Part model, mm, in its own coordinate system. A direction names the side the tool comes from. Coordinates: 2 decimals unless noted, no trailing zeros. Loops run counter-clockwise (first coordinate to the right, second up) from the corner with the lowest first, then second, coordinate; pieces in that order, holes last.
```python
from build123d import *

# Parameters (mm, degrees)
CROQUIS1_R              = 2.4
SALIENTE_EXTRUIR1_DEPTH = 6
CROQUIS2_R              = 3.5
SALIENTE_EXTRUIR2_DEPTH = 1
CROQUIS3_R              = 18.5
SALIENTE_EXTRUIR3_DEPTH = 3
CORTAR_EXTRUIR1_DEPTH   = 2
CROQUIS5_R              = 2.075
CORTAR_EXTRUIR2_DEPTH   = 2.2
CROQUIS6_R              = 1.25
CORTAR_EXTRUIR3_DEPTH   = 28.300915736


with BuildPart() as part:
    # Croquis1 → Saliente-Extruir1 (new body)
    with BuildSketch(Plane.XY):
        Circle(CROQUIS1_R)
    extrude(amount=SALIENTE_EXTRUIR1_DEPTH)

    # Croquis2 → Saliente-Extruir2 (add)
    with BuildSketch(Plane(origin=(0, 0, 0), x_dir=(-1, 0, 0), z_dir=(0, 0, -1))):
        Circle(CROQUIS2_R)
    extrude(amount=SALIENTE_EXTRUIR2_DEPTH)

    # Croquis3 → Saliente-Extruir3 (add)
    with BuildSketch(Plane(origin=(0, 0, -1), x_dir=(-1, 0, 0), z_dir=(0, 0, -1))):
        Circle(CROQUIS3_R)
    extrude(amount=SALIENTE_EXTRUIR3_DEPTH)

    # Croquis4 → Cortar-Extruir1 (cut)
    with BuildSketch(Plane(origin=(0, 0, -4), x_dir=(-1, 0, 0), z_dir=(0, 0, -1))):
        with BuildLine():
            Line((0, 15.331093131), (-1.68173019, 12.418250997))
            ThreePointArc((-1.68173019, 12.418250997), (-1.649800286, 12.176683613), (-1.408167444, 12.145252908))
            ThreePointArc((-1.408167444, 12.145252908), (-0.72912408, 12.427844555), (0, 12.524467551))
            ThreePointArc((0, 12.524467551), (0.72912408, 12.427844555), (1.408167444, 12.145252908))
            ThreePointArc((1.408167444, 12.145252908), (1.649800286, 12.176683613), (1.68173019, 12.418250997))
            Line((1.68173019, 12.418250997), (0, 15.331093131))
        make_face()
    extrude(amount=-CORTAR_EXTRUIR1_DEPTH, mode=Mode.SUBTRACT)

    # Croquis5 → Cortar-Extruir2 (cut)
    with BuildSketch(Plane.XY.offset(6)):
        Circle(CROQUIS5_R)
    extrude(amount=-CORTAR_EXTRUIR2_DEPTH, mode=Mode.SUBTRACT)

    # Croquis6 → Cortar-Extruir3 (cut, through all)
    with BuildSketch(Plane.XY.offset(3.8)):
        Circle(CROQUIS6_R)
    extrude(amount=-CORTAR_EXTRUIR3_DEPTH, mode=Mode.SUBTRACT)


solid = part.part
```
Q1. Saw through at D-D (x = 5.5). List the corners of the cut face in (y, z), plus the area to 3 significant figures.
Q2. Probe line 1 (Y direction, x = 0, z = 4.7) (3 decimals); line 2 (Y direction, x = 0, z = 1.5); line 3 (Z direction, x = 2.5, y = -15.5). List the from-to ranges inside material, lowest first.
Q3. Saw through at A-A (y = 0). List the corners of the cut face in (x, z) (3 decimals).
Q4. Tool access for faces 1 (the flat face through (0.829, 13.895, -3.014)), 2 (the cylindrical face through (-0.27, -1.22, -0.05)), 3 (the cylindrical face through (1.29, 2.024, 2.958)): list every direction of +Z, -Z, +X, -X, +Y, -Y with a clear straight run to the whole face (end or side of a thin tool).
Q5. Drop flat-ended pins along their axis: P1, Ø1.5, axis at y = -5.5, z = 1.5, coming from the -X side; P2, Ø1, axis at y = 6, z = -2, coming from the +X side; P3, Ø3.5, axis at x = 0, y = 0, coming from the +Z side; P4, Ø2, axis at y = 2.5, z = 3.5, coming from the +X side. Give the stop position or say it passes through.
Q6. Mould opens along X. For faces 4 (the flat face through (-0.853, 13.854, -3.014)), 5 (the flat face through (0, 13, -2)), 6 (the cylindrical face through (-3.233, -1.341, -0.493)), 7 (the flat face through (0, -4, -4)) say: released by +X, released by -X, zero draft, split by the parting line, or undercut.
Q7. Saw through at B-B (z = 0.75). List the corners of the cut face in (x, y), plus the area to 3 significant figures.
Q8. Saw through at C-C (y = -6). List the corners of the cut face in (x, z).
Checked values:
1. outline: (-17.66, -4) - (17.66, -4) - (17.66, -1) - (-17.66, -1) - close
1. area: 106 mm2
2. line 1: y = -2.4 to -2.075, 2.075 to 2.4
2. line 2: y = -2.4 to -1.25, 1.25 to 2.4
2. line 3: z = -4 to -1
3. outline: (-18.5, -4) - (-1.25, -4) - (-1.25, 3.8) - (-2.075, 3.8) - (-2.075, 6) - (-2.4, 6) - (-2.4, 0) - (-3.5, 0) - (-3.5, -1) - (-18.5, -1) - close; (1.25, -4) - (18.5, -4) - (18.5, -1) - (3.5, -1) - (3.5, 0) - (2.4, 0) - (2.4, 6) - (2.075, 6) - (2.075, 3.8) - (1.25, 3.8) - close
4. face 1: -Z
4. face 2: +Z, -Z
4. face 3: +Z
5. P1: passes through
5. P2: stops at x = 17.66
5. P3: stops at z = 3.8
5. P4: stops at x = 1.87
6. face 4: undercut
6. face 5: undercut
6. face 6: split by the parting line
6. face 7: zero draft
7. outline: circle Ø4.8 at (0, 0); hole circle Ø2.5 at (0, 0)
7. area: 13.2 mm2
8. outline: (-17.5, -4) - (17.5, -4) - (17.5, -1) - (-17.5, -1) - close
